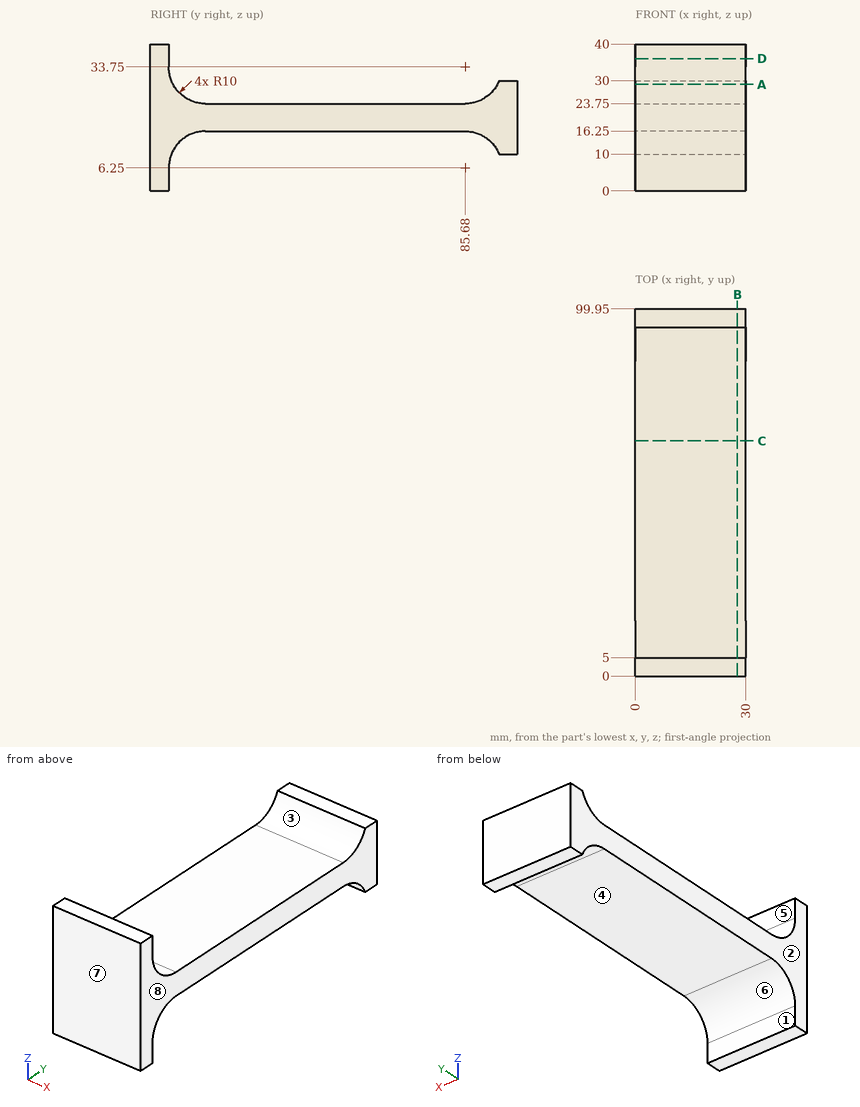
Geometry: see drawing. Coordinates: mm, zero at the bounding-box minimum. A direction names the side the tool comes from. Coordinates: 2 decimals unless noted, no trailing zeros. Order: outer loops, then holes, each group sorted by start corner. A loop starts at its lowest first (then second) coordinate and runs counter-clockwise, first axis right, second up. Notation, with made-up numbers: M 74.25,77.5 L 131.25,77.5 A17 ccw 131.25,89.5 Z; hole C 8,85 d8. An arc over 180 degrees is marked long. Answer in a Markdown table with one row per item. Add a question column.
Q1. Section query A-A on z = 29. Return the cut outline in (x, y).
Q2. Reachability of the marked faces 1, 2, 3 and 4 from +Z, -Z, +X, -X, +Y, -Y: full face, straight path, thin tool, end or side. Return the list, or none.
Q3. Line query: L1, parallel to Z at x = 10.75, y = 68; L2, parallel to Y at x = 9.75, z = 34; L3, parallel to Y at x = 11.75, z = 29. Output: solid intervals per line, ascending.
Q4. Contact query for flat-ended pins moving along their axis: P1, Ø2, axis at x = 20.5, y = 18, coming from the -Z side; P2, Ø5, axis at x = 26, z = 4, coming from the +Y side; P3, Ø1.5, axis at x = 10, y = 97, coming from the -Z side. Output: stop coordinate, or through.
Q5. Section query D-D on z = 36. Return the cut outline in (x, y).
Q6. Mould query, pull axis Y, two halves, no side actions, for the marked faces 5, 6, 7 and 8. Classes: released by +Y, released by -Y, zero draft, split by the parting line, or undercut.
Q7. Section query C-C on y = 64. Return the cut outline in (x, z), and give its area (3 significant figures).
Q8. Section query B-B on x = 27.75. Return the cut outline in (y, z).
Completed:
| question | item | result |
|---|---|---|
| 1 | outline | M 0,0 L 30,0 L 30,6.2 L 0,6.2 Z; M 0,94.48 L 30,94.48 L 30,99.95 L 0,99.95 Z |
| 2 | face 1 | -Z, +X, -X, +Y |
| 2 | face 2 | +Z, -Z, -X, +Y, -Y |
| 2 | face 3 | +Z, +X, -X |
| 2 | face 4 | -Z, +X, -X |
| 3 | L1 | z = 16.25 to 23.75 |
| 3 | L2 | y = 0 to 5 |
| 3 | L3 | y = 0 to 6.2, 94.48 to 99.95 |
| 4 | P1 | stops at z = 16.25 |
| 4 | P2 | stops at y = 5 |
| 4 | P3 | stops at z = 10 |
| 5 | outline | M 0,0 L 30,0 L 30,5 L 0,5 Z |
| 6 | face 5 | released by +Y |
| 6 | face 6 | undercut |
| 6 | face 7 | released by -Y |
| 6 | face 8 | zero draft |
| 7 | outline | M 0,16.25 L 30,16.25 L 30,23.75 L 0,23.75 Z |
| 7 | area | 225 mm2 |
| 8 | outline | M 0,0 L 5,0 L 5,6.25 A10 cw 15,16.25 L 85.68,16.25 A10 cw 94.95,10 L 99.95,10 L 99.95,30 L 94.95,30 A10 cw 85.68,23.75 L 15,23.75 A10 cw 5,33.75 L 5,40 L 0,40 Z |
